from build123d import *

# Parameters (mm, degrees)
BOSS_EXTRUDE1_DEPTH = 3


with BuildPart() as part:
    # Sketch1 → Boss-Extrude1 (new body)
    with BuildSketch(Plane(origin=(0, 0, 0), x_dir=(1, 0, 0), z_dir=(0, 1, 0))):
        Polygon((22.079481216, 3.028725772), (16.079481216, 3.028725772), (16.079481216, 7.528725772), (0.079481216, 7.528725772), (0.079481216, 3.028725772), (-5.920518784, 3.028725772), (6.579481216, -11.971274228), (6.579481216, -8.971274228), (9.579481216, -8.971274228), (9.579481216, -11.971274228), align=None)
        Polygon((15.674356378, 0.028725772), (0.484606054, 0.028725772), (5.484606054, -5.971274228), (10.674356378, -5.971274228), align=None, mode=Mode.SUBTRACT)
    extrude(amount=BOSS_EXTRUDE1_DEPTH)


solid = part.part
Source: CAD feature listing. Evaluate the final solid. Frame: model axes, mm. A direction names the side the tool comes from. Round coordinates to 2 decimals unless told otherwise and drop trailing zeros. Loops run counter-clockwise (first coordinate to the right, second up) from the corner with the lowest first, then second, coordinate; pieces in that order, holes last. Notation, with made-up numbers: (-21.75, 76) -> (13.25, 76) arc R29 cw to (13.25, 98) -> close; hole circle Ø9 at (65.5, -37.75). An arc over 180 degrees is marked (long way). Answer as a JSON object with one key per item and string values. Group by question number.
Q1. Section query B-B (y = 2.4). Output: boundary loops of the cut face in (x, z), plus the area to 3 significant figures.
Q2. Access query for faces 1 (the flat face through (16.079, 1, -5)), 2 (the flat face through (13.14, 1.48, 3.01)), 3 (the flat face through (8, 3, -2)), 4 (the flat face through (-3, 1, -3.029)), 5 (the flat face through (6.579, 1, 10)). Directions: +Z, -Z, +X, -X, +Y, -Y. A direction counts if a zero-diameter tool reaches every point of the face in a straight line with its end or side. Return the directions, or none.
Q3. Ray query, line 1 (X direction, y = 2.8, z = -5.5); line 2 (Z direction, x = 8, y = 0.35); line 3 (Z direction, x = 0.75, y = 0.75). Return the intervals inside material, ascending. Write a range as from..to.
Q4. Section query C-C (z = 2.5). Output: boundary loops of the cut face in (x, y), plus the area to 3 significant figures.
Q5. Mould query, pull axis Z, two halves, no side actions, for faces 6 (the flat face through (0.242, 1.479, 4.366)), 7 (the flat face through (8, 0, -2)), 8 (the flat face through (8, 1, 5.971)). Classes: pulls with the +Z half, pulls with the -Z half, needs draft (parallel to the pull), parting line crosses it, or undercut.
Q6. Section query D-D (x = -1). Output: boundary loops of the cut face in (y, z).
Q7. Contact query for flat-ended pins moving along their axis: P1, Ø1, axis at y = 1.5, z = 7, coming from the +X side; P2, Ø0.9, axis at y = 1, z = -5, coming from the +X side; P3, Ø0.9, axis at y = 1, z = -4.5, coming from the -X side; P4, Ø5, axis at x = 10.5, z = 2, coming from the +Y side. Output: stop coordinate, or through.
Q8. Section query A-A (x = 8.5). Output: boundary loops of the cut face in (y, z).
Completed:
{
 "1": {"outline": "(-5.92, -3.03) -> (0.08, -3.03) -> (0.08, -7.53) -> (16.08, -7.53) -> (16.08, -3.03) -> (22.08, -3.03) -> (9.58, 11.97) -> (9.58, 8.97) -> (6.58, 8.97) -> (6.58, 11.97) -> close; hole (0.48, -0.03) -> (15.67, -0.03) -> (10.67, 5.97) -> (5.48, 5.97) -> close", "area": "234 mm²"},
 "2": {"face 1": "-Z, +X, +Y, -Y", "face 2": "+Y, -Y", "face 3": "+Z, -Z, +X, -X, +Y", "face 4": "-Z, -X, +Y, -Y", "face 5": "+Z, +Y, -Y"},
 "3": {"line 1": "0.08..16.08", "line 2": "-7.53..-0.03, 5.97..8.97", "line 3": "-7.53..-0.03, 0.29..4.98"},
 "4": {"outline": "(-1.31, 0) -> (2.59, 0) -> (2.59, 3) -> (-1.31, 3) -> close; (13.57, 0) -> (17.47, 0) -> (17.47, 3) -> (13.57, 3) -> close", "area": "23.4 mm²"},
 "5": {"face 6": "pulls with the +Z half", "face 7": "needs draft", "face 8": "undercut"},
 "6": {"outline": "(0, -3.03) -> (3, -3.03) -> (3, 2.88) -> (0, 2.88) -> close"},
 "7": {"P1": "x = 14.14", "P2": "x = 16.08", "P3": "x = 0.08", "P4": "y = 3"},
 "8": {"outline": "(0, -7.53) -> (3, -7.53) -> (3, -0.03) -> (0, -0.03) -> close; (0, 5.97) -> (3, 5.97) -> (3, 8.97) -> (0, 8.97) -> close"}
}
